from build123d import *

# Parameters (mm, degrees)
F0_R     = 15.9
F1_DEPTH = 10
F3_DEPTH = 10
F4_R     = 5
F5_DEPTH = 10
F6_R     = 25
F6_R_2   = 15.9
F7_DEPTH = 50
F8_W     = 7.1
F8_H     = 12
F9_DEPTH = 25


with BuildPart() as f1:
    # F0 (on Top) → F1 (new body)
    with BuildSketch(Plane.XY):
        with BuildLine():
            ThreePointArc((42.6098881125, -68.8390092879), (28.7369466924, -36.2564924246), (24.9782102729, -1.0435571688))
            ThreePointArc((24.9782102729, -1.0435571688), (0, 25), (-24.9782102729, -1.0435571688))
            ThreePointArc((-24.9782102729, -1.0435571688), (-28.7369466924, -36.2564924246), (-42.6098881125, -68.8390092879))
            ThreePointArc((-42.6098881125, -68.8390092879), (0, -145), (42.6098881125, -68.8390092879))
        make_face()
        with Locations((0, -95)):
            Circle(F0_R, mode=Mode.SUBTRACT)
    extrude(amount=-F1_DEPTH)

    # F2 (on Top) → F3 (cut, through all)
    with BuildSketch(Plane.XY):
        with BuildLine():
            Line((-11, 0), (-11, -45))
            ThreePointArc((-11, -45), (0, -56), (11, -45))
            Line((11, -45), (11, 0))
            ThreePointArc((11, 0), (0, 11), (-11, 0))
        make_face()
    extrude(amount=-F3_DEPTH, mode=Mode.SUBTRACT)

    # F4 (on face) → F5 (cut, through all)
    with BuildSketch(Plane.XY):
        with Locations((-35, -95)):
            Circle(F4_R)
        with Locations((-24.7487373415, -119.7487373415)):
            Circle(F4_R)
        with Locations((0, -130)):
            Circle(F4_R)
        with Locations((24.7487373415, -119.7487373415)):
            Circle(F4_R)
        with Locations((35, -95)):
            Circle(F4_R)
    extrude(amount=-F5_DEPTH, mode=Mode.SUBTRACT)

    # F6 (on face) → F7 (join)
    with BuildSketch(Plane.XY):
        with Locations((0, -95)):
            Circle(F6_R)
        with Locations((0, -95)):
            Circle(F6_R_2, mode=Mode.SUBTRACT)
    extrude(amount=F7_DEPTH)

    # F8 (on Right) → F9 (cut, symmetric)
    with BuildSketch(Plane.YZ):
        with Locations((-95, 44)):
            Rectangle(F8_W, F8_H)
    extrude(amount=F9_DEPTH, both=True, mode=Mode.SUBTRACT)


solid = f1.part
Model file for the job. Use its own axes, mm. A direction names the side the tool comes from. Coordinates: 2 decimals unless noted, no trailing zeros. Order: outer loops, then holes, each group sorted by start corner. A loop starts at its lowest first (then second) coordinate and runs counter-clockwise, first axis right, second up. Notation, with made-up numbers: (-24, 18) -> (23, 18) arc R30 cw to (23, 45) -> close; hole circle Ø3 at (-8.5, -25). An arc over 180 degrees is marked (long way). Return JSON: item names as keys, results as strings. Group by question number.
Item 1: Wall check: line 1 along Y through (x, z) = (0, 7); line 2 along X through (y, z) = (-92, -6.5); line 3 along X through (y, z) = (-1, -4.5). Give the ranges that are in metal, low to high. Write a range as [from, to].
Item 2: Saw through at A-A on y = -123. Write the cut outline in (x, z), then the cut area to 3 significant figures.
Item 3: Flat gauge pins, fed straight in: P1, Ø3, axis at x = 8, z = 38.5, coming from the -Y side; P2, Ø10, axis at x = -19.5, z = 45.5, coming from the +Y side; P3, Ø12, axis at x = 21, z = 1, coming from the +Y side. Where does each tip first touch, or does it go through?
Item 4: Tool access for faces 4 (the flat face through (0, -112, 50)), 5 (the cylindrical face through (0, -56, -5)), 6 (the flat face through (-1, -78, -10)), 7 (the flat face through (20, -95, 38)), 8 (the cylindrical face through (23.09, -104.58, 24.65)): list every direction of +Z, -Z, +X, -X, +Y, -Y with a clear straight run to the whole face (end or side of a thin tool).
Item 5: Saw through at D-D on z = 35. Write the cut outline in (x, y), then the cut area to 3 significant figures.
Item 6: Saw through at B-B on x = 0. Write the cut outline in (y, z).
Item 7: Saw through at C-C on x = 32. Write the cut outline in (y, z), then the cut area to 3 significant figures.
Item 8: Pull direction X, two halves, no side cores. Call faces 1 (the flat face through (-11, -22, -5)), 2 (the cylindrical face through (-28.61, -35.77, -4.93)), 3 (the flat face through (-20, -95, 38)): pulls with the +X half, pulls with the -X half, needs draft (parallel to the pull), parting line crosses it, or undercut.
Values found:
{
 "1": {"line 1": "y = [-120, -110.9], [-79.1, -70]", "line 2": "x = [-49.91, -39], [-31, -15.61], [15.61, 31], [39, 49.91]", "line 3": "x = [-24.98, -11], [11, 24.98]"},
 "2": {"outline": "(-41.42, -10) -> (-28.55, -10) -> (-28.55, 0) -> (-41.42, 0) -> close; (-20.95, -10) -> (20.95, -10) -> (20.95, 0) -> (-20.95, 0) -> close; (28.55, -10) -> (41.42, -10) -> (41.42, 0) -> (28.55, 0) -> close", "area": "677 mm2"},
 "3": {"P1": "stops at y = -119.14", "P2": "stops at y = -74.63", "P3": "stops at y = 19.94"},
 "4": {"face 4": "+Z, +X, -X, +Y, -Y", "face 5": "+Z, -Z", "face 6": "-Z, +X, -X, +Y, -Y", "face 7": "+Z, +X, -X", "face 8": "+Z"},
 "5": {"outline": "circle Ø50 at (0, -95); hole circle Ø31.8 at (0, -95)", "area": "1,170 mm2"},
 "6": {"outline": "(-145, -10) -> (-135, -10) -> (-135, 0) -> (-145, 0) -> close; (-125, -10) -> (-110.9, -10) -> (-110.9, 50) -> (-120, 50) -> (-120, 0) -> (-125, 0) -> close; (-79.1, -10) -> (-56, -10) -> (-56, 0) -> (-70, 0) -> (-70, 50) -> (-79.1, 50) -> close; (11, -10) -> (25, -10) -> (25, 0) -> (11, 0) -> close"},
 "7": {"outline": "(-133.42, -10) -> (-99, -10) -> (-99, 0) -> (-133.42, 0) -> close; (-91, -10) -> (-46.79, -10) -> (-46.79, 0) -> (-91, 0) -> close", "area": "786 mm2"},
 "8": {"face 1": "undercut", "face 2": "pulls with the -X half", "face 3": "needs draft"}
}
